Autodesk Inventor part; units mm, degrees
ref_plane "YZ Plane" through (0, 0, 0) normal (1, 0, 0) x (0, 1, 0)
ref_plane "XZ Plane" through (0, 0, 0) normal (0, 1, 0) x (-1, 0, 0)
ref_plane "XY Plane" through (0, 0, 0) normal (0, 0, 1) x (1, 0, 0)
sketch "Skizze1" plane through (0, 0, 0) normal (0, 0, 1) x (1, 0, 0)
  line L0 (0, 0) -> (52, 0)
  line L1 (0, 0) -> (0, 3)
  line L2 (0, 3) -> (6, 3)
  line L3 (6, 3) -> (6, 5)
  line L4 (6, 5) -> (52, 5)
  line L5 (52, 5) -> (52, 0)
  dimension "d1" = 6
  dimension "d2" = 10
  dimension "d3" = 6
  dimension "d18" = 52
revolve "Umdrehung1" add sketch "Skizze1" angle 360 about axis through (0, 0, 0) along (1, 0, 0)
sketch "Skizze2" plane through (52, 0, 0) normal (1, 0, 0) x (0, 0, -1)
  point P0 (0, 0)
  point P1 (0, 0)
hole "Bohrung1" at (52, 0, 0) direction (-1, 0, 0) diameter 4.917 depth 13 tip angle 118
thread "Gewinde1"
properties part number "kicker_mitte_alt" material "Aluminium 6061"
Geometry: final body of the model. Coordinates: model frame, mm. A direction names the side the tool comes from. Round coordinates to 2 decimals unless told otherwise and drop trailing zeros. Order: outer loops, then holes, each group sorted by start corner. A loop starts at its lowest first (then second) coordinate and runs counter-clockwise, first axis right, second up. Notation, with made-up numbers: (51.5, 51.25) -> (55.5, 51.25) arc R29 cw to (55.5, 87.25) -> close; hole circle Ø7 at (43.25, 36). An arc over 180 degrees is marked (long way). Use one line per item in the form item = value.
(1) Access query for faces 1 (the face through (6, 3.3, 0.1)), 2 (the face through (29.32, -1.08, -4.88)). Directions: +Z, -Z, +X, -X, +Y, -Y. A direction counts if a zero-diameter tool reaches every point of the face in a straight line with its end or side. Return the directions, or none.
Results list:
face_1 = -X
face_2 = +X, -X
(2) Ray query, probe 1 along Z at (x, y) = (42, 0); probe 2 along X at (y, z) = (-1, -3); probe 3 along Y at (x, z) = (14, -4). Return the intervals inside material, ascending. Write a range as [from, to].
Results list:
probe_1 = [-5, -2.46], [2.46, 5]
probe_2 = [6, 52]
probe_3 = [-3, 3]
(3) First-contact query: pin 1 Ø3 at (y, z) = (0, 0) entering from -X; pin 2 Ø1.5 at (x, z) = (7.5, -2.5) entering from -Y; pin 3 Ø1 at (x, y) = (27, -3.5) entering from +Z. Flat tips, straight axial feed; report the tip coordinate or a pass-through.
Results list:
pin_1 = 0
pin_2 = -4.68
pin_3 = 4
(4) Section B-B on z = 4.5. Return loops of the section in (x, y).
Results list:
outline = (6, -2.18) -> (52, -2.18) -> (52, 2.18) -> (6, 2.18) -> close
(5) Draft query along Y for faces 3 (the face through (45.409, -0.738, -2.345)), 4 (the face through (3, -3, 0)), 5 (the face through (52, 2, -2)). Return one class per face: pulls with the +Y half, pulls with the -Y half, needs draft (parallel to the pull), parting line crosses it, or undercut.
Results list:
face_3 = undercut
face_4 = parting line crosses it
face_5 = needs draft
(6) Section A-A on x = 8. Return loops of the section in (y, z).
Results list:
outline = circle Ø10 at (0, 0)
